Could you check a few things on this drawing? It's one solid part, dimensions in mm from its lowest x, y, z. A direction names the side the tool comes from. Coordinates: 2 decimals unless noted, no trailing zeros. Write each loop counter-clockwise with the first axis right and the second up, starting at its lowest first coordinate (ties: lowest second). Pieces come first, ordered by that corner, then holes. Notation, with made-up numbers: (26.25, 69) - (73.25, 69) arc R19 ccw to (73.25, 81) - close; hole circle Ø8 at (-21.5, 53.5). An arc over 180 degrees is marked (long way). Write item = value, one per line. Start each with the question number.
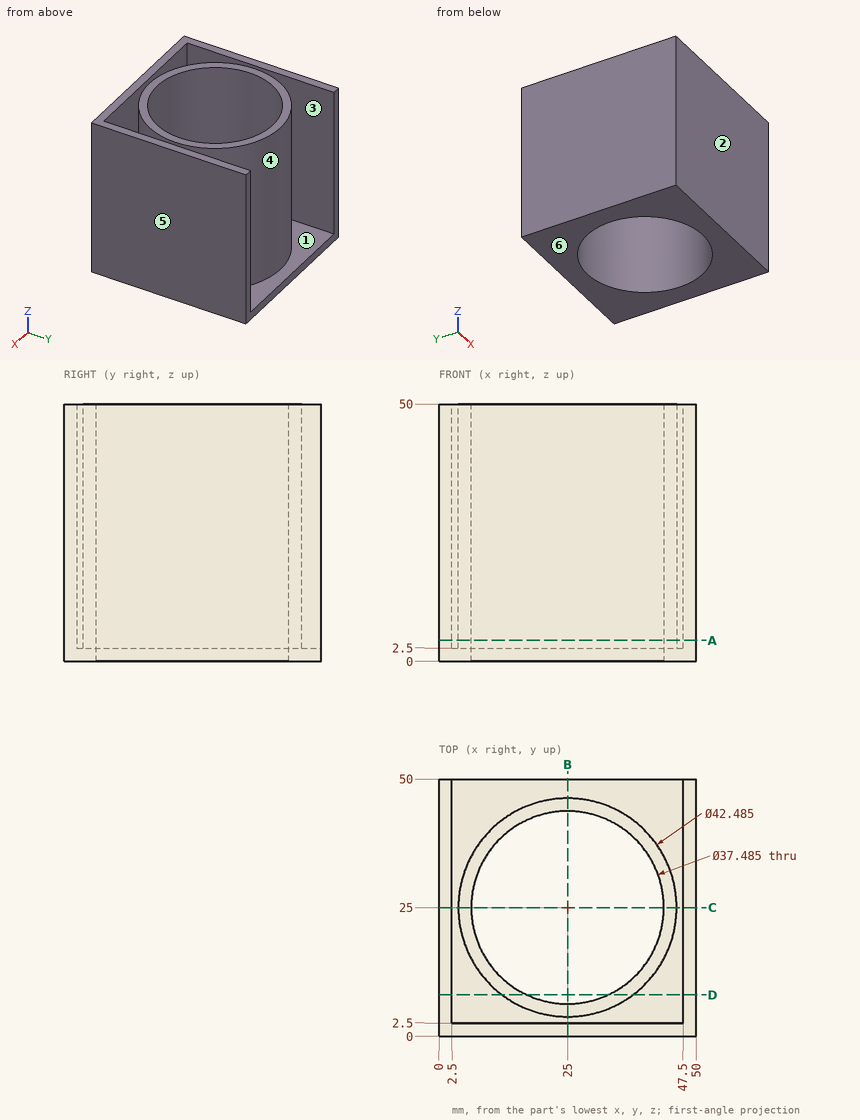
1) Suppose I cut it at C-C on y = 25. Please give me the cut outline in (x, z).
2) Suppose I cut it at A-A on z = 4. Please give me the cut outline in (x, y) (1 decimal).
3) Thinking about a two-plate mould opening in X: for the marked faces 4, 5 and 6, which applies, +X half, -X half, draft (parallel to the pull), parting line (faces both ways), or undercut?
4) For P1, Ø1.5, axis at x = 7, z = 9.5, coming from the +Y side; P2, Ø13.5, axis at x = 18.5, z = 28, coming from the +Y side; P3, Ø12, axis at x = 12.5, y = 34, coming from the -Z side, each with a flat end and sliding along its axis, tell me the tip position at first contact or that it passes through.
5) If I drill on probe 1 along Y at (x, z) = (25, 11); probe 2 along Y at (x, z) = (13.5, 7); probe 3 along X at (y, z) = (23, 39), over which ranges is the centre line in solid material (lowest first)? Write a range as [from, to].
6) Which directions (+Z, -Z, +X, -X, +Y, -Y) give clear straight access to the entire face, cutting with the end or side of a thin tool? Please do the marked faces 1, 2 and 3.
7) Suppose I cut it at D-D on y = 8. Please give me the cut outline in (x, z).
8) Suppose I cut it at B-B on x = 25. Please give me the cut outline in (y, z), plus the area to 3 significant figures.
Reply:
q1.outline = (0, 0) - (6.26, 0) - (6.26, 50) - (3.76, 50) - (3.76, 2.5) - (2.5, 2.5) - (2.5, 50) - (0, 50) - close; (43.74, 0) - (50, 0) - (50, 50) - (47.5, 50) - (47.5, 2.5) - (46.24, 2.5) - (46.24, 50) - (43.74, 50) - close
q2.outline = (0, 0) - (50, 0) - (50, 50) - (47.5, 50) - (47.5, 2.5) - (2.5, 2.5) - (2.5, 50) - (0, 50) - close; circle Ø42.5 at (25, 25); hole circle Ø37.5 at (25, 25)
q3.face_4 = undercut
q3.face_5 = +X half
q3.face_6 = draft
q4.P1 = 37.4
q4.P2 = 46.24
q4.P3 = 0
q5.probe_1 = [0, 2.5], [3.76, 6.26], [43.74, 46.24]
q5.probe_2 = [0, 2.5], [7.14, 10.2], [39.8, 42.86]
q5.probe_3 = [0, 2.5], [3.85, 6.36], [43.64, 46.15], [47.5, 50]
q6.face_1 = +Z
q6.face_2 = +Z, -Z, +X, -X, -Y
q6.face_3 = +Z, +Y
q7.outline = (0, 0) - (17.11, 0) - (17.11, 50) - (12.26, 50) - (12.26, 2.5) - (2.5, 2.5) - (2.5, 50) - (0, 50) - close; (32.89, 0) - (50, 0) - (50, 50) - (47.5, 50) - (47.5, 2.5) - (37.74, 2.5) - (37.74, 50) - (32.89, 50) - close
q8.outline = (0, 0) - (6.26, 0) - (6.26, 50) - (3.76, 50) - (3.76, 2.5) - (2.5, 2.5) - (2.5, 50) - (0, 50) - close; (43.74, 0) - (50, 0) - (50, 2.5) - (46.24, 2.5) - (46.24, 50) - (43.74, 50) - close
q8.area = 388 mm^2
